The listing builds one solid part. Answer for the finished solid, in the listing's coordinates (mm). Round coordinates to 2 decimals unless told otherwise and drop trailing zeros. Write each loop counter-clockwise with the first axis right and the second up, starting at its lowest first coordinate (ties: lowest second). Pieces come first, ordered by that corner, then holes. Notation, with made-up numbers: M 0.5,43.25 L 22.5,43.25 A29 ccw 22.5,80.25 Z; hole C 32.25,79.5 d10. An arc over 180 degrees is marked long. Write each question's results on one line, items separated by ' | '.
from build123d import *

# Parameters (mm, degrees)
BOSS_EXTRUDE1_DEPTH = 1.5
SKETCH5_R           = 1.6
CUT_EXTRUDE2_DEPTH  = 3.5
CUT_EXTRUDE4_DEPTH  = 10


with BuildPart() as part:
    # Sketch2 → Boss-Extrude1 (new body)
    with BuildSketch(Plane.XY):
        Polygon((803.47776474, 117.914742868), (586.414001465, 117.914742868), (578.414001465, 109.914742868), (578.414001465, -2.5), (586.414001465, -10.5), (828.47776474, -10.5), (828.47776474, 92.914742868), align=None)
        Polygon((613.414001465, 102.914742868), (613.414001465, 4.5), (600.414001465, 4.5), (590.414001465, 14.5), (590.414001465, 92.914742868), (600.414001465, 102.914742868), align=None, mode=Mode.SUBTRACT)
        Polygon((793.47776474, 4.5), (816.47776474, 4.5), (816.47776474, 87.94418012), (801.507201992, 102.914742868), (793.47776474, 102.914742868), align=None, mode=Mode.SUBTRACT)
    extrude(amount=BOSS_EXTRUDE1_DEPTH)

    # Sketch5 → Cut-Extrude2 (cut)
    with BuildSketch(Plane.XY.offset(1.5)):
        with Locations((588.414001465, 111.914742868)):
            Circle(SKETCH5_R)
        with Locations((588.414001465, -4.5)):
            Circle(SKETCH5_R)
        with Locations((818.47776474, -4.5)):
            Circle(SKETCH5_R)
        with Locations((623.414001465, 111.914742868)):
            Circle(SKETCH5_R)
        with Locations((623.414001465, -4.5)):
            Circle(SKETCH5_R)
        with Locations((800.992483366, 111.914742868)):
            Circle(SKETCH5_R)
        with Locations((818.47776474, 94.429461494)):
            Circle(SKETCH5_R)
        with Locations((800.992483366, -4.5)):
            Circle(SKETCH5_R)
    extrude(amount=-CUT_EXTRUDE2_DEPTH, mode=Mode.SUBTRACT)

    # Sketch6 → Cut-Extrude4 (cut)
    with BuildSketch(Plane.XY.offset(1.5)):
        Polygon((658.469461081, 102.914742868), (644.327325457, 102.914742868), (629.059768774, 87.647186185), (629.059768774, 73.505050562), align=None)
        Polygon((686.751596705, 102.914742868), (672.609461081, 102.914742868), (629.059768774, 59.365050562), (629.059768774, 45.222914938), align=None)
        Polygon((715.033732329, 102.914742868), (700.891596705, 102.914742868), (629.059768774, 31.082914938), (629.059768774, 16.940779314), align=None)
        Polygon((743.315867952, 102.914742868), (729.173732329, 102.914742868), (630.75898946, 4.5), (644.901125084, 4.5), align=None)
        Polygon((771.598003576, 102.914742868), (757.455867952, 102.914742868), (659.041125084, 4.5), (673.183260708, 4.5), align=None)
        Polygon((773.47776474, 76.512368409), (773.47776474, 90.654504032), (687.323260708, 4.5), (701.465396331, 4.5), align=None)
        Polygon((773.47776474, 48.230232785), (773.47776474, 62.372368409), (715.605396331, 4.5), (729.747531955, 4.5), align=None)
        Polygon((773.47776474, 19.948097161), (773.47776474, 34.090232785), (743.887531955, 4.5), (758.029667579, 4.5), align=None)
    extrude(amount=-CUT_EXTRUDE4_DEPTH, mode=Mode.SUBTRACT)


solid = part.part
1) The mould has two halves that part along Y. Classify faces 1 (the face through (582.358, -6.444, 0.74)), 2 (the face through (816.15, 105.24, 0.74)), 3 (the face through (595.484, 9.43, 0.74)): +Y half, -Y half, draft (parallel to the pull), parting line (faces both ways), or undercut.
Return value:
face 1: -Y half | face 2: +Y half | face 3: undercut
2) Section C-C (x = 648) is taken. Determine the outline of the cut face in (y, z), then the cut area to 3 significant figures.
Return value:
outline: M -10.5,0 L 7.6,0 L 7.6,1.5 L -10.5,1.5 Z; M 21.74,0 L 35.88,0 L 35.88,1.5 L 21.74,1.5 Z; M 50.02,0 L 64.16,0 L 64.16,1.5 L 50.02,1.5 Z; M 78.31,0 L 92.45,0 L 92.45,1.5 L 78.31,1.5 Z; M 102.91,0 L 117.91,0 L 117.91,1.5 L 102.91,1.5 Z | area: 113 mm²
3) Section A-A (x = 608) is taken. Determine the outline of the cut face in (y, z), then the cut area to 3 significant figures.
Return value:
outline: M -10.5,0 L 4.5,0 L 4.5,1.5 L -10.5,1.5 Z; M 102.91,0 L 117.91,0 L 117.91,1.5 L 102.91,1.5 Z | area: 45.0 mm²
4) Section B-B (y = 38.5) is taken. State how many separate pieces and enclosed holes the cut face has, then the cut area to 3 significant figures.
Return value:
separate pieces: 8 | enclosed holes: 0 | area: 200 mm²
5) Each of these flat-tipped pins is pushed along its axis until it touches: pin 1 (6 mm diameter, centred on x = 740, y = 50.5, fed in from -Z); pin 2 (0.8 mm diameter, centred on x = 808.5, z = 1, fed in from +Y). Where does it stop, or does it pass through?
Return value:
pin 1: through | pin 2: y = 113.29
6) Find the intervals of material crossed by line 1 (Y direction, x = 746.5, z = 0.3); line 2 (Y direction, x = 632, z = 0.65); line 3 (Y direction, x = 799, z = 0.9), in increasing order.
Return value:
line 1: -10.5 to 4.5, 7.11 to 21.25, 35.39 to 49.53, 63.68 to 77.82, 91.96 to 117.91 | line 2: -10.5 to 4.5, 5.74 to 19.88, 34.02 to 48.16, 62.31 to 76.45, 90.59 to 117.91 | line 3: -10.5 to 4.5, 102.91 to 117.91
